from build123d import *

# Parameters (mm, degrees)
SKETCH1_R           = 2.4
BOSS_EXTRUDE1_DEPTH = 14
SKETCH3_W           = 16.77722104
SKETCH3_H           = 8
CUT_EXTRUDE2_DEPTH  = 26
SKETCH4_R           = 2.5
SKETCH4_R_2         = 1.5
BOSS_EXTRUDE2_DEPTH = 7.54


with BuildPart() as part:
    # Sketch1 → Boss-Extrude1 (new body)
    with BuildSketch(Plane(origin=(0, 0, 0), x_dir=(1, 0, 0), z_dir=(0, 1, 0))):
        with BuildLine():
            Line((-12.125, 7.5), (-12.125, -7.5))
            Line((-12.125, -7.5), (1.066020546, -3.725483216))
            ThreePointArc((1.066020546, -3.725483216), (3.875, 0), (1.066020546, 3.725483216))
            Line((1.066020546, 3.725483216), (-12.125, 7.5))
        make_face()
        with Locations(Location((0, 0, 0), (0, 0, 270))):
            Circle(SKETCH1_R, mode=Mode.SUBTRACT)
    extrude(amount=BOSS_EXTRUDE1_DEPTH)

    # Sketch3 → Cut-Extrude2 (cut, symmetric)
    with BuildSketch(Plane.XY):
        with Locations((-1.73638948, 7)):
            Rectangle(SKETCH3_W, SKETCH3_H)
    extrude(amount=CUT_EXTRUDE2_DEPTH, both=True, mode=Mode.SUBTRACT)

    # Sketch4 → Boss-Extrude2 (add)
    # profile 1 of 2: a face of its own
    with BuildSketch(Plane.ZY.offset(12.125)):
        with Locations(Location((4, 7, 0), (0, 0, 180))):
            Circle(SKETCH4_R)
        with Locations((4, 7)):
            Circle(SKETCH4_R_2, mode=Mode.SUBTRACT)
    # profile 2 of 2: a face of its own
    with BuildSketch(Plane.ZY.offset(12.125)):
        with Locations(Location((-4, 7, 0), (0, 0, 180))):
            Circle(SKETCH4_R)
        with Locations((-4, 7)):
            Circle(SKETCH4_R_2, mode=Mode.SUBTRACT)
    extrude(amount=BOSS_EXTRUDE2_DEPTH)


solid = part.part
Source: CAD feature listing. Evaluate the final solid. Frame: model axes, mm. A direction names the side the tool comes from. Round coordinates to 2 decimals unless told otherwise and drop trailing zeros. Loops run counter-clockwise (first coordinate to the right, second up) from the corner with the lowest first, then second, coordinate; pieces in that order, holes last. Notation, with made-up numbers: M 68,14 L 118,14 A15 cw 118,32 Z; hole C -33.75,-27.5 d2. An arc over 180 degrees is marked long. Return JSON: item names as keys, results as strings. Group by question number.
1. Pin query (flat end, axial travel): pin 1 (3 mm diameter, centred on x = 0, z = 0, fed in from -Y); pin 2 (2.5 mm diameter, centred on y = 7, z = -4, fed in from -X) (3 decimals); pin 3 (3 mm diameter, centred on x = -16, z = -4, fed in from +Y); pin 4 (1.8 mm diameter, centred on y = 7, z = 4, fed in from +X) (3 decimals). Return the tip coordinate at first contact, or that it passes through.
2. Section query A-A on y = 13. Output: boundary loops of the cut face in (x, z) (3 decimals), and give its area (3 significant figures).
3. Section query D-D on x = -17. Output: boundary loops of the cut face in (y, z), and give its area (3 significant figures).
4. Reachability of faces 4 (the face through (3.874, 12.479, 0.07)), 5 (the face through (-10.125, 7, 0)), 6 (the face through (-12.125, 7, 0)) from +Z, -Z, +X, -X, +Y, -Y: full face, straight path, thin tool, end or side. Return the list, or none.
5. Section query B-B on x = -2.75. Output: boundary loops of the cut face in (y, z).
6. Material intervals for line 1 along Y through (x, z) = (-17.5, -4); line 2 along Y through (x, z) = (-3, -2.5); line 3 along X through (y, z) = (1, 0) (3 decimals), sorted ascending. Write a range as from..to.
7. Mould query, pull axis X, two halves, no side actions, for faces 1 (the face through (-15.842, 5.536, -4.325)), 2 (the face through (2.024, 1.479, 1.29)), 3 (the face through (-12.125, 7, -4)). Classes: released by +X, released by -X, zero draft, split by the parting line, or undercut.
8. Section query C-C on z = -0.25. Output: boundary loops of the cut face in (x, y) (3 decimals), and give its area (3 significant figures).
Checks:
{
 "1": {"pin 1": "passes through", "pin 2": "stops at x = -12.125", "pin 3": "stops at y = 9.5", "pin 4": "stops at x = -10.125"},
 "2": {"outline": "M -12.125,-7.5 L 1.066,-3.725 A3.875 ccw 1.066,3.725 L -12.125,7.5 Z; hole C 0,0 d4.8", "area": "145 mm²"},
 "3": {"outline": "C 7,-4 d5; C 7,4 d5; hole C 7,-4 d3; hole C 7,4 d3", "area": "25.1 mm²"},
 "4": {"face 4": "+X, +Y, -Y", "face 5": "+Z, -Z, +X", "face 6": "-X"},
 "5": {"outline": "M 0,-4.82 L 3,-4.82 L 3,4.82 L 0,4.82 Z; M 11,-4.82 L 14,-4.82 L 14,4.82 L 11,4.82 Z"},
 "6": {"line 1": "y = 4.5..5.5, 8.5..9.5", "line 2": "y = 0..3, 11..14", "line 3": "x = -12.125..-2.4, 2.4..3.875"},
 "7": {"face 1": "zero draft", "face 2": "undercut", "face 3": "released by -X"},
 "8": {"outline": "M -12.125,0 L -2.387,0 L -2.387,3 L -10.125,3 L -10.125,11 L -2.387,11 L -2.387,14 L -12.125,14 Z; M 2.387,0 L 3.867,0 L 3.867,3 L 2.387,3 Z; M 2.387,11 L 3.867,11 L 3.867,14 L 2.387,14 Z", "area": "83.3 mm²"}
}
